Geometry check sheet. Reference: the model listing, model coordinates, mm. A direction names the side the tool comes from. Round coordinates to 2 decimals unless told otherwise and drop trailing zeros. Loops run counter-clockwise (first coordinate to the right, second up) from the corner with the lowest first, then second, coordinate; pieces in that order, holes last. Notation, with made-up numbers: (6, 89) -> (60, 89) arc R17 cw to (60, 103) -> close; hole circle Ø9 at (83, 40). An arc over 180 degrees is marked (long way). Use a Markdown table: item, result. Add a question column.
Q1. Set-up check for faces 1 (the face through (-10.1, -4.73, -8.44)), 2 (the face through (9, -6, 2.5)), 3 (the face through (0, 6, -10)), 4 (the face through (-8, -10, 4)): record each of +Z, -Z, +X, -X, +Y, -Y from which the full face is reachable in a straight line by a thin tool's end or side.
Q2. Sectioned sample at D-D, the plane z = -9. Enter the section's corners in (x, y).
Q3. Sectioned sample at B-B, the plane x = 12.5. Enter the section's corners in (y, z).
Q4. Release check for a two-part mould opening along Y. For faces 5 (the face through (15, 6, 5)), 6 (the face through (-0.1, 9.5, 10.2)), 7 (the face through (9, -2.9, -4)), 8 (the face through (-0.903, -5.613, -8.049)) record: released by +Y, released by -Y, zero draft, split by the parting line, or undercut.
Q5. Sectioned sample at A-A, the plane y = 7. Enter the section's corners in (x, z).
Q6. Sectioned sample at C-C, the plane x = 8. Enter the section's corners in (y, z).
Q7. Material ranges on L1, parallel to Z at x = 12, y = -9.75; L2, parallel to Y at x = 3.5, z = -9.25; L3, parallel to Y at x = 10, z = -3, recorded low to high.
Q8. Gauge pin test, flat ends, axial feed: P1, Ø0.8, axis at y = -6, z = 4, coming from the -X side; P2, Ø3, axis at x = -3.5, y = -5.73, coming from the -Z side; P3, Ø0.8, axis at y = -7, z = -3.5, coming from the +X side. Record the tip position at first contact, or that the pin passes through.
```python
from build123d import *

# Parameters (mm, degrees)
SKETCH4_W           = 32
SKETCH4_H           = 23
BOSS_EXTRUDE3_DEPTH = 9.5
SKETCH5_W           = 29
SKETCH5_H           = 20
CUT_EXTRUDE2_DEPTH  = 8
SKETCH7_W           = 10
SKETCH7_H           = 7
CUT_EXTRUDE4_DEPTH  = 36.305806888
SKETCH8_W           = 32
SKETCH8_H           = 23
BOSS_EXTRUDE4_DEPTH = 10
SKETCH12_R          = 2.6
CUT_EXTRUDE5_DEPTH  = 7
CIRPATTERN1_COUNT   = 2
CIRPATTERN1_ANGLE   = 180
SKETCH13_W          = 15
SKETCH13_H          = 2.791622882
CUT_EXTRUDE6_DEPTH  = 7.1
SKETCH14_W          = 32
SKETCH14_H          = 23
BOSS_EXTRUDE5_DEPTH = 5


with BuildPart() as part:
    # Sketch4 → Boss-Extrude3 (new body)
    with BuildSketch(Plane(origin=(0, 0, 0), x_dir=(1, 0, 0), z_dir=(0, 1, 0))):
        Rectangle(SKETCH4_W, SKETCH4_H)
    extrude(amount=BOSS_EXTRUDE3_DEPTH)

    # Sketch5 → Cut-Extrude2 (cut)
    with BuildSketch(Plane(origin=(0, 9.5, 0), x_dir=(1, 0, 0), z_dir=(0, 1, 0))):
        Rectangle(SKETCH5_W, SKETCH5_H)
    extrude(amount=-CUT_EXTRUDE2_DEPTH, mode=Mode.SUBTRACT)

    # Sketch7 → Cut-Extrude4 (cut, through all)
    with BuildSketch(Plane(origin=(16, 0, 0), x_dir=(0, 0, -1), z_dir=(1, 0, 0))):
        with Locations((0, 6)):
            Rectangle(SKETCH7_W, SKETCH7_H)
    extrude(amount=-CUT_EXTRUDE4_DEPTH, mode=Mode.SUBTRACT)

    # Sketch8 → Boss-Extrude4 (add)
    with BuildSketch(Plane(origin=(0, 0, 0), x_dir=(-1, 0, 0), z_dir=(0, -1, 0))):
        Rectangle(SKETCH8_W, SKETCH8_H)
    extrude(amount=BOSS_EXTRUDE4_DEPTH)

    # Sketch12 → Cut-Extrude5 (cut)
    with BuildSketch(Plane(origin=(0, 0, -11.5), x_dir=(-1, 0, 0), z_dir=(0, 0, -1))):
        with Locations((-12.5, -5.726898225)):
            Circle(SKETCH12_R)
        with Locations(Location((-3.5, -5.726898225, 0), (0, 0, 180))):
            Circle(SKETCH12_R)
        with Locations((3.5, -5.726898225)):
            Circle(SKETCH12_R)
        with Locations(Location((12.5, -5.726898225, 0), (0, 0, 180))):
            Circle(SKETCH12_R)
    cut_extrude5 = extrude(amount=-CUT_EXTRUDE5_DEPTH, mode=Mode.SUBTRACT)

    # CirPattern1: Cut-Extrude5 ×2 about axis
    cirpattern1_axis = Axis((0, 1.5, 0), (0, -1, 0))
    for i in range(1, CIRPATTERN1_COUNT):
        add(cut_extrude5.rotate(cirpattern1_axis, i * CIRPATTERN1_ANGLE / (CIRPATTERN1_COUNT - 1)), mode=Mode.SUBTRACT)

    # Sketch13 → Cut-Extrude6 (cut)
    with BuildSketch(Plane(origin=(0, -10, 0), x_dir=(-1, 0, 0), z_dir=(0, -1, 0))):
        with Locations((8.5, 3.895811441)):
            Rectangle(SKETCH13_W, SKETCH13_H)
        with Locations((-8.5, 3.895811441)):
            Rectangle(SKETCH13_W, SKETCH13_H)
        with Locations((-8.5, -3.895811441)):
            Rectangle(SKETCH13_W, SKETCH13_H)
        with Locations((8.5, -3.895811441)):
            Rectangle(SKETCH13_W, SKETCH13_H)
    extrude(amount=-CUT_EXTRUDE6_DEPTH, mode=Mode.SUBTRACT)

    # Sketch14 → Boss-Extrude5 (add)
    with BuildSketch(Plane(origin=(0, -10, 0), x_dir=(-1, 0, 0), z_dir=(0, -1, 0))):
        Rectangle(SKETCH14_W, SKETCH14_H)
    extrude(amount=BOSS_EXTRUDE5_DEPTH)


solid = part.part
```
Values:
| question | item | result |
|---|---|---|
| 1 | face 1 | -Z |
| 1 | face 2 | +X |
| 1 | face 3 | +Y |
| 1 | face 4 | -X |
| 2 | outline | (-16, -15) -> (16, -15) -> (16, 9.5) -> (14.5, 9.5) -> (14.5, 1.5) -> (-14.5, 1.5) -> (-14.5, 9.5) -> (-16, 9.5) -> close; hole circle Ø5.2 at (-12.5, -5.73); hole circle Ø5.2 at (-3.5, -5.73); hole circle Ø5.2 at (3.5, -5.73); hole circle Ø5.2 at (12.5, -5.73) |
| 3 | outline | (-15, -11.5) -> (-8.33, -11.5) -> (-8.33, -5.29) -> (-10, -5.29) -> (-10, -2.5) -> (-2.9, -2.5) -> (-2.9, -5.29) -> (-3.13, -5.29) -> (-3.13, -11.5) -> (9.5, -11.5) -> (9.5, -10) -> (1.5, -10) -> (1.5, 10) -> (9.5, 10) -> (9.5, 11.5) -> (-3.13, 11.5) -> (-3.13, 5.29) -> (-2.9, 5.29) -> (-2.9, 2.5) -> (-10, 2.5) -> (-10, 5.29) -> (-8.33, 5.29) -> (-8.33, 11.5) -> (-15, 11.5) -> close |
| 4 | face 5 | zero draft |
| 4 | face 6 | released by +Y |
| 4 | face 7 | undercut |
| 4 | face 8 | undercut |
| 5 | outline | (-16, -11.5) -> (16, -11.5) -> (16, -5) -> (14.5, -5) -> (14.5, -10) -> (-14.5, -10) -> (-14.5, -5) -> (-16, -5) -> close; (-16, 5) -> (-14.5, 5) -> (-14.5, 10) -> (14.5, 10) -> (14.5, 5) -> (16, 5) -> (16, 11.5) -> (-16, 11.5) -> close |
| 6 | outline | (-15, -11.5) -> (9.5, -11.5) -> (9.5, -10) -> (1.5, -10) -> (1.5, 10) -> (9.5, 10) -> (9.5, 11.5) -> (-15, 11.5) -> close; hole (-10, -5.29) -> (-2.9, -5.29) -> (-2.9, -2.5) -> (-10, -2.5) -> close; hole (-10, 2.5) -> (-2.9, 2.5) -> (-2.9, 5.29) -> (-10, 5.29) -> close |
| 7 | L1 | -11.5 to -5.29, -2.5 to 2.5, 5.29 to 11.5 |
| 7 | L2 | -15 to -8.33, -3.13 to 1.5 |
| 7 | L3 | -15 to -10, -2.9 to 1.5 |
| 8 | P1 | x = -1 |
| 8 | P2 | z = -2.5 |
| 8 | P3 | x = 1 |
